Geometry check sheet. Reference: the model listing, model coordinates, mm. A direction names the side the tool comes from. Coordinates: 2 decimals unless noted, no trailing zeros. Write each loop counter-clockwise with the first axis right and the second up, starting at its lowest first coordinate (ties: lowest second). Pieces come first, ordered by that corner, then holes. Notation, with made-up numbers: (89, -20) -> (128, -20) arc R25 cw to (128, -7) -> close; hole circle Ø8 at (88.25, 4). An arc over 180 degrees is marked (long way). Answer as CSV lines item,"result".
```python
from build123d import *

# Parameters (mm, degrees)
BOSS_EXTRUDE1_DEPTH = 1.6
CUT_EXTRUDE1_DEPTH  = 43.927962915
SKETCH4_R           = 1.375
CUT_EXTRUDE2_DEPTH  = 43.927962915


with BuildPart() as part:
    # Sketch1 → Boss-Extrude1 (new body)
    with BuildSketch(Plane.XY):
        with BuildLine():
            Line((-29.5, -28), (29.5, -28))
            ThreePointArc((29.5, -28), (31.621320344, -27.121320344), (32.5, -25))
            Line((32.5, -25), (32.5, 25))
            ThreePointArc((32.5, 25), (31.621320344, 27.121320344), (29.5, 28))
            Line((29.5, 28), (-29.5, 28))
            ThreePointArc((-29.5, 28), (-31.621320344, 27.121320344), (-32.5, 25))
            Line((-32.5, 25), (-32.5, 9.5))
            ThreePointArc((-32.5, 9.5), (-32.207106781, 8.792893219), (-31.5, 8.5))
            Line((-31.5, 8.5), (-28.5, 8.5))
            ThreePointArc((-28.5, 8.5), (-27.792893219, 8.207106781), (-27.5, 7.5))
            Line((-27.5, 7.5), (-27.5, -7.5))
            ThreePointArc((-27.5, -7.5), (-27.792893219, -8.207106781), (-28.5, -8.5))
            Line((-28.5, -8.5), (-31.5, -8.5))
            ThreePointArc((-31.5, -8.5), (-32.207106781, -8.792893219), (-32.5, -9.5))
            Line((-32.5, -9.5), (-32.5, -25))
            ThreePointArc((-32.5, -25), (-31.621320344, -27.121320344), (-29.5, -28))
        make_face()
    extrude(amount=BOSS_EXTRUDE1_DEPTH)

    # Sketch3 → Cut-Extrude1 (cut, through all)
    with BuildSketch(Plane.XY.offset(1.6)):
        with BuildLine():
            Line((13.5, -8.5), (13.5, -24.5))
            ThreePointArc((13.5, -24.5), (12.5, -25.5), (11.5, -24.5))
            Line((11.5, -24.5), (11.5, -8.5))
            ThreePointArc((11.5, -8.5), (12.5, -7.5), (13.5, -8.5))
        make_face()
    extrude(amount=-CUT_EXTRUDE1_DEPTH, mode=Mode.SUBTRACT)

    # Sketch4 → Cut-Extrude2 (cut, through all)
    with BuildSketch(Plane.XY.offset(1.6)):
        with Locations((-29, 24.5)):
            Circle(SKETCH4_R)
        with Locations((29, 24.5)):
            Circle(SKETCH4_R)
        with Locations(Location((29, -24.5, 0), (0, 0, 180))):
            Circle(SKETCH4_R)
        with Locations(Location((-29, -24.5, 0), (0, 0, 180))):
            Circle(SKETCH4_R)
    extrude(amount=-CUT_EXTRUDE2_DEPTH, mode=Mode.SUBTRACT)


solid = part.part
```
Item 1: Release check for a two-part mould opening along Y. For faces 4 (the cylindrical face through (31.64, 27.1, 0.79)), 5 (the flat face through (-32.5, 17, 1)), 6 (the flat face through (-27.5, 0, 1)), 7 (the cylindrical face through (-31.64, -27.1, 0.79)) record: +Y half, -Y half, draft (parallel to the pull), parting line (faces both ways), or undercut.
Responses:
face 4,"+Y half"
face 5,"draft"
face 6,"undercut"
face 7,"-Y half"
Item 2: Thickness scan on probe 1 along Y at (x, z) = (29, 0.4) (3 decimals); probe 2 along X at (y, z) = (-24.5, 0.7) (3 decimals); probe 3 along Y at (x, z) = (-29, 1.25) (3 decimals). Record the ranges inside material, lowest first.
Responses:
probe 1,"y = -28 to -25.875, -23.125 to 23.125, 25.875 to 28"
probe 2,"x = -32.5 to -30.375, -27.625 to 11.5, 13.5 to 27.625, 30.375 to 32.5"
probe 3,"y = -28 to -25.875, -23.125 to -8.5, 8.5 to 23.125, 25.875 to 28"
Item 3: Cross-section at C-C, the plane y = -5. Record the cut outline in (x, z).
Responses:
outline,"(-27.5, 0) -> (32.5, 0) -> (32.5, 1.6) -> (-27.5, 1.6) -> close"
Item 4: Cross-section at A-A, the plane x = 12.5. Record the cut outline in (y, z), plus the area to 3 significant figures.
Responses:
outline,"(-28, 0) -> (-25.5, 0) -> (-25.5, 1.6) -> (-28, 1.6) -> close; (-7.5, 0) -> (28, 0) -> (28, 1.6) -> (-7.5, 1.6) -> close"
area,"60.8 mm2"
Item 5: Depth check by flat-ended pin: pin 1 Ø0.8 at (x, z) = (-30.5, 1) entering from -Y; pin 2 Ø2 at (x, y) = (-29, 24.5) entering from +Z; pin 3 Ø0.8 at (y, z) = (1, 1) entering from -X. Enter the tip coordinate at first touch or a pass-through.
Responses:
pin 1,"stops at y = -27.94"
pin 2,"passes through"
pin 3,"stops at x = -27.5"
Item 6: Set-up check for faces 1 (the flat face through (-30, 8.5, 1)), 2 (the flat face through (11.5, -17, 1)), 3 (the flat face through (0, -28, 1)): record each of +Z, -Z, +X, -X, +Y, -Y from which the full face is reachable in a straight line by a thin tool's end or side.
Responses:
face 1,"+Z, -Z, -X"
face 2,"+Z, -Z"
face 3,"+Z, -Z, +X, -X, -Y"
Item 7: Cross-section at B-B, the plane z = 1.3. Record the cut outline in (x, y) (3 decimals), plus the area to 3 significant figures.
Responses:
outline,"(-32.5, -25) arc R3 ccw to (-29.5, -28) -> (29.5, -28) arc R3 ccw to (32.5, -25) -> (32.5, 25) arc R3 ccw to (29.5, 28) -> (-29.5, 28) arc R3 ccw to (-32.5, 25) -> (-32.5, 9.5) arc R1 ccw to (-31.5, 8.5) -> (-28.5, 8.5) arc R1 cw to (-27.5, 7.5) -> (-27.5, -7.5) arc R1 cw to (-28.5, -8.5) -> (-31.5, -8.5) arc R1 ccw to (-32.5, -9.5) -> close; hole circle Ø2.75 at (-29, -24.5); hole circle Ø2.75 at (-29, 24.5); hole (11.5, -24.5) arc R1 ccw to (13.5, -24.5) -> (13.5, -8.5) arc R1 ccw to (11.5, -8.5) -> close; hole circle Ø2.75 at (29, -24.5); hole circle Ø2.75 at (29, 24.5)"
area,"3,490 mm2"
